```python
from build123d import *

# Parameters (mm, degrees)
SKETCH2_W                = 82.31886
SKETCH2_H                = 38.6207
BOSS_EXTRUDE1_DEPTH      = 3.175
BOSS_EXTRUDE2_DEPTH      = 25.4
BOSS_EXTRUDE2_DEPTH_BACK = 3.175
SKETCH3_W                = 3.175
SKETCH3_H                = 38.6207
SKETCH4_R                = 0.561869351
SKETCH4_R_2              = 0.521667109
SKETCH4_R_3              = 0.606918095
SKETCH4_R_4              = 0.92346357
CUT_EXTRUDE1_DEPTH       = 94.276837661
M3_CLEARANCE_HOLE1_D     = 3.6


with BuildPart() as part:
    # Sketch2 → Boss-Extrude1 (new body)
    with BuildSketch(Plane.XY):
        with Locations((37.34943, 15.50035)):
            Rectangle(SKETCH2_W, SKETCH2_H)
    extrude(amount=BOSS_EXTRUDE1_DEPTH)

    # Sketch3 → Boss-Extrude2 (add, two sides: drawn at the far end of the back side and taken through both)
    with BuildSketch(Plane.XY.offset(3.175).offset(-BOSS_EXTRUDE2_DEPTH_BACK)):
        with Locations((-5.3975, 15.50035)):
            Rectangle(SKETCH3_W, SKETCH3_H)
        with Locations((80.09636, 15.50035)):
            Rectangle(SKETCH3_W, SKETCH3_H)
        Polygon((78.50886, -3.81), (-3.81, -3.81), (-6.985, -3.81), (-6.985, -6.985), (81.68386, -6.985), (81.68386, -3.81), align=None)
    extrude(amount=BOSS_EXTRUDE2_DEPTH + BOSS_EXTRUDE2_DEPTH_BACK)

    # Sketch4 → Cut-Extrude1 (cut, through all)
    with BuildSketch(Plane(origin=(0, 0, 0), x_dir=(-1, 0, 0), z_dir=(0, 0, -1))):
        with Locations((-26.682215, 25.41285)):
            Circle(SKETCH4_R)
        with Locations((-3.682215, 25.41285)):
            Circle(SKETCH4_R_2)
        with Locations((-26.682215, 2.41285)):
            Circle(SKETCH4_R_3)
        with Locations((-3.682215, 2.41285)):
            Circle(SKETCH4_R_4)
        with Locations((-48.016645, 2.41285)):
            Circle(SKETCH4_R_3)
        with Locations((-71.016645, 2.41285)):
            Circle(SKETCH4_R_4)
        with Locations((-71.016645, 25.41285)):
            Circle(SKETCH4_R_2)
        with Locations((-48.016645, 25.41285)):
            Circle(SKETCH4_R)
    extrude(amount=-CUT_EXTRUDE1_DEPTH, mode=Mode.SUBTRACT)

    # M3 Clearance Hole1 (through all)
    with Locations(Plane(origin=(0, 0, 0), x_dir=(-1, 0, 0), z_dir=(0, 0, -1))):
        with Locations((-71.016645, 25.41285), (-71.016645, 2.41285), (-3.682215, 2.41285), (-26.682215, 2.41285), (-48.016645, 2.41285), (-48.016645, 25.41285), (-26.682215, 25.41285), (-3.682215, 25.41285)):
            Hole(M3_CLEARANCE_HOLE1_D / 2)


solid = part.part
```
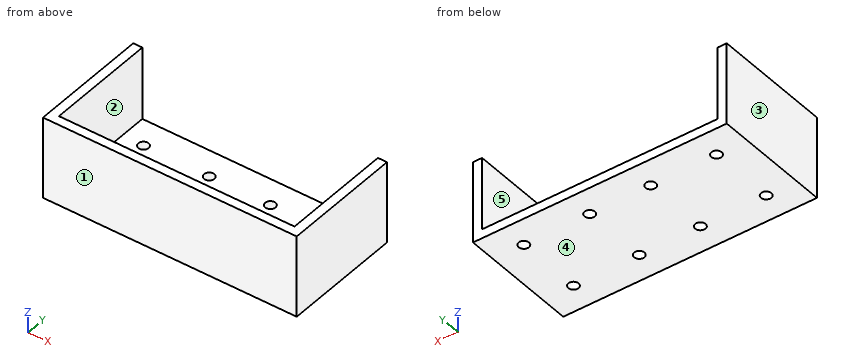
Can you work these out from the model? Positions are in its coordinate system, mm. Face numbers are marked on the shaded views. A direction names the side the tool comes from. Coordinates: 2 decimals unless noted, no trailing zeros. Loops run counter-clockwise (first coordinate to the right, second up) from the corner with the lowest first, then second, coordinate; pieces in that order, holes last. Notation, with made-up numbers: (84, 27.25) - (96, 27.25) arc R16 ccw to (96, 47.25) - close; hole circle Ø9 at (73, -40). An arc over 180 degrees is marked (long way). Answer as CSV lines item,"result". Start each with the question number.
1) Suppose I cut it at B-B (x = 52). Please give me the cut outline in (y, z) (3 decimals).
2) Which directions (+Z, -Z, +X, -X, +Y, -Y) give clear straight access to the entire face, cutting with the end or side of a thin tool? Please do the marked faces 1 and 2.
3) Thinking about a two-plate mould opening in X: for the marked faces 3, 4 and 5, which applies, pulls with the +X half, pulls with the -X half, needs draft (parallel to the pull), parting line crosses it, or undercut?
4) For pin 1 (12.5 mm diameter, centred on x = 30.5, z = 9.5, fed in from +Y); pin 2 (4.5 mm diameter, centred on x = 26.68, y = 25.41, fed in from +Z) (3 decimals), each with a flat end and sliding along its axis, tell me the tip position at first contact or that it passes through.
5) Suppose I cut it at A-A (y = 1.5). Please give me the cut outline in (x, z) (3 decimals).
6) Suppose I cut it at D-D (y = 7.5). Please give me the cut outline in (x, z) (3 decimals).
7) I need wall thicknesses on line 1 (X direction, y = 32.5, z = 24.25) (3 decimals); line 2 (Y direction, x = 19, z = 5.5) (3 decimals); line 3 (Z direction, x = 63.5, y = 26.5) (3 decimals). Which ranges of each line are inside material? Lowest first, please. Write a range as from..to.
8) Suppose I cut it at C-C (z = 12.25). Please give me the cut outline in (x, y) (3 decimals), plus the area to 3 significant figures.
Check result:
1,outline,"(-6.985, 0) - (34.811, 0) - (34.811, 3.175) - (-3.81, 3.175) - (-3.81, 28.575) - (-6.985, 28.575) - close"
2,face 1,"+Z, -Z, +X, -X, -Y"
2,face 2,"+Z, +Y"
3,face 3,"pulls with the -X half"
3,face 4,"needs draft"
3,face 5,"undercut"
4,pin 1,"stops at y = -3.81"
4,pin 2,"stops at z = 3.175"
5,outline,"(-6.985, 0) - (2.131, 0) - (2.131, 3.175) - (-3.81, 3.175) - (-3.81, 28.575) - (-6.985, 28.575) - close; (5.234, 0) - (25.131, 0) - (25.131, 3.175) - (5.234, 3.175) - close; (28.234, 0) - (46.465, 0) - (46.465, 3.175) - (28.234, 3.175) - close; (49.568, 0) - (69.465, 0) - (69.465, 3.175) - (49.568, 3.175) - close; (72.568, 0) - (81.684, 0) - (81.684, 28.575) - (78.509, 28.575) - (78.509, 3.175) - (72.568, 3.175) - close"
6,outline,"(-6.985, 0) - (81.684, 0) - (81.684, 28.575) - (78.509, 28.575) - (78.509, 3.175) - (-3.81, 3.175) - (-3.81, 28.575) - (-6.985, 28.575) - close"
7,line 1,"x = -6.985..-3.81, 78.509..81.684"
7,line 2,"y = -6.985..-3.81"
7,line 3,"z = 0..3.175"
8,outline,"(-6.985, -6.985) - (81.684, -6.985) - (81.684, 34.811) - (78.509, 34.811) - (78.509, -3.81) - (-3.81, -3.81) - (-3.81, 34.811) - (-6.985, 34.811) - close"
8,area,"527 mm²"
